Design review of the part built by this model. Coordinates are the model's own, in mm. A direction names the side the tool comes from. Coordinates: 2 decimals unless noted, no trailing zeros. Write each loop counter-clockwise with the first axis right and the second up, starting at its lowest first coordinate (ties: lowest second). Pieces come first, ordered by that corner, then holes. Notation, with made-up numbers: (44.25, 19.25) - (66.25, 19.25) arc R16 ccw to (66.25, 41.25) - close; hole circle Ø6 at (52, -20). An arc over 180 degrees is marked (long way). One line per item, written item: value.
Autodesk Inventor part; units mm, degrees
ref_plane "Arbeitsebene1" through (53.5, 2, 88) normal (1, 0, 0) x (0, 0, -1)
ref_plane "Arbeitsebene7" through (18, 0, -130) normal (0, 0, -1) x (-1, 0, 0)
ref_plane "YZ Plane" through (0, 0, 0) normal (1, 0, 0) x (0, 1, 0)
sketch "Skizze1" plane through (0, 0, 0) normal (0, 1, 0) x (-1, 0, 0)
  line L0 (53, 90) -> (53, 20)
  line L1 (53, 20) -> (18, 0)
  line L2 (18, 0) -> (-18, 0)
  line L3 (-18, 0) -> (-53, 20)
  line L4 (-53, 20) -> (-53, 90)
  line L5 (-53, 90) -> (-39.5, 90)
  line L6 (-39.5, 90) -> (-39.5, 30)
  line L7 (-39.5, 30) -> (-15, 15)
  line L8 (-15, 15) -> (15, 15)
  line L9 (15, 15) -> (39.5, 30)
  line L10 (39.5, 30) -> (39.5, 90)
  line L11 (39.5, 90) -> (53, 90)
  line L12 (0, -234) -> (0, 144) construction
  point P0 (0, 0)
  dimension "d0" = 79
  dimension "d1" = 13.5
  dimension "d2" = 13.5
  dimension "d3" = 90
  dimension "d5" = 60
  dimension "d6" = 15
  dimension "d7" = 60
  dimension "d8" = 70
  dimension "d9" = 70
  dimension "d12" = 15
  dimension "d13" = 15
  dimension "d14" = 18
  dimension "d15" = 18
extrude "Extrusion1" add sketch "Skizze1" along normal blind 20
sketch "Skizze2" plane through (18, 0, 0) normal (0, 0, -1) x (-1, 0, 0)
  line L0 (57.5, 20) -> (33, 20) construction
  line L1 (8.5, 0) -> (27.5, 0)
  line L2 (27.5, 0) -> (27.5, 20)
  line L3 (27.5, 20) -> (8.5, 20)
  line L4 (8.5, 20) -> (8.5, 0)
  line L5 (18, -4) -> (18, 24) construction
  line L6 (0, 0) -> (36, 0) construction
  point P0 (18, 0)
  point P1 (18, 0)
  point P2 (18, 20)
  dimension "d75" = 19
extrude "Extrusion2" add sketch "Skizze2" along normal blind 180
ref_plane "Arbeitsebene1" through (53.5, 2, 88) normal (1, 0, 0) x (0, 0, -1)
sketch "Skizze3" plane through (53, 0, 90) normal (1, 0, 0) x (0, 0, -1)
  line L0 (0, 10) -> (14, 10) construction
  line L1 (0, 0) -> (0, 20) construction
  circle A0 centre (14, 10) radius 6
  dimension "d44" = 14
  dimension "d87" = 12
extrude "Extrusion3" cut sketch "Skizze3" against normal through all
ref_plane "Arbeitsebene5" through (18, 0, -160) normal (0, 0, -1) x (-1, 0, 0)
ref_plane "Arbeitsebene6" through (18, 0, -100) normal (0, 0, -1) x (-1, 0, 0)
ref_plane "Arbeitsebene7" through (18, 0, -130) normal (0, 0, -1) x (-1, 0, 0)
sketch "Skizze13" plane through (9.5, 0, 0) normal (1, 0, 0) x (0, 0, -1)
  line L0 (160, 24) -> (160, -4) construction
  line L1 (100, 24) -> (100, -4) construction
  line L2 (180, 0) -> (180, 20) construction
  line L3 (180, 10) -> (100, 10) construction
  point P0 (0, 0)
  point P1 (160, 10)
hole "Bohrung2" at (9.5, 10, -100) at (9.5, 10, -160) direction (-1, 0, 0) diameter 8.376 end through all
sketch "Skizze11" plane through (0, 20, 0) normal (0, 1, 0) x (1, 0, 0)
  line L0 (9.5, 0) -> (18, 0)
  line L1 (18, 0) -> (18, 61.5)
  line L2 (9.5, 70) -> (9.5, 0)
  line L3 (-9.5, 0) -> (-9.5, 180)
  line L4 (-9.5, 0) -> (-18, 0)
  line L5 (-18, 0) -> (-18, 61.5)
  line L6 (-9.5, 70) -> (-9.5, 0)
  arc A0 (9.5, 70) -> (18, 61.5) centre (18, 70) ccw
  arc A1 (-18, 61.5) -> (-9.5, 70) centre (-18, 70) ccw
  point P0 (0, 0)
  point P1 (-9.5, 70)
  dimension "d80" = 70
  dimension "d81" = 70
extrude "Extrusion7" add sketch "Skizze11" against normal up to surface (20 mm away)
sketch "Skizze12" plane through (18, 0, -180) normal (0, 0, -1) x (-1, 0, 0)
  line L0 (27.5, 20) -> (8.5, 20) construction
  point P0 (18, 0)
  dimension "Gabel_FixierungPart_Width" = 19
chamfer "Fase1" distance 1.25 angle 45 4 edges at (9.5, 10, -155.812) (9.5, 10, -95.812) (-9.5, 10, -155.812) (-9.5, 10, -95.812)
chamfer "Fase2" distance 0.5 angle 45 4 edges at (53, 10, 82) (39.5, 10, 82) (-53, 10, 82) (-39.5, 10, 82)
equation "\"d1\" = d2"
equation "\"d75\" = ParallelMecha_Contact_Dist - 2 * Gabel_FixationShaft_Contact_Thickness"
equation "\"d81\" = d80"
equation "\"Fixation_dist2\" = -Total_Bearing_Hole_Dist"
properties part number "Adaptationhorizontalachse" material "Aluminum 6061-AHC"
1. Wall thickness on line 1 along Y through (x, z) = (-49, 76); line 2 along Y through (x, z) = (-4, -160); line 3 along X through (y, z) = (3, -82): over which ranges is each line inside the solid? List them lowest first.
Answer block:
line 1: y = 0 to 4, 16 to 20
line 2: y = 0 to 5.81, 14.19 to 20
line 3: x = -9.5 to 9.5
2. Consider section D-D, the plane z = -73. Write out the cut boundary in (x, y).
Answer block:
outline: (-9.5, 0) - (9.5, 0) - (9.5, 20) - (-9.5, 20) - close
3. Consider section B-B, the plane z = 76. Write out the cut boundary in (x, y).
Answer block:
outline: (-53, 0) - (-39.5, 0) - (-39.5, 3.5) - (-40, 4) - (-52.5, 4) - (-53, 3.5) - close; (-53, 16.5) - (-52.5, 16) - (-40, 16) - (-39.5, 16.5) - (-39.5, 20) - (-53, 20) - close; (39.5, 0) - (53, 0) - (53, 3.5) - (52.5, 4) - (40, 4) - (39.5, 3.5) - close; (39.5, 16.5) - (40, 16) - (52.5, 16) - (53, 16.5) - (53, 20) - (39.5, 20) - close
4. Mouldability with a two-part tool opening along X and no side actions: class faces 4 (the face through (-39.5, 10, 60)), 5 (the face through (-18, 10, -30)), 6 (the face through (-27.078, 9.86, 22.395)), 7 (the face through (46, 10, 82)) as released by +X, released by -X, zero draft, split by the parting line, or undercut.
Answer block:
face 4: undercut
face 5: released by -X
face 6: undercut
face 7: zero draft
5. For faces 1 (the face through (9.5, 10, -124)), 2 (the face through (39.5, 10, 60)), 3 (the face through (4, 0, -24)), list the 3-axis set-ups (+Z, -Z, +X, -X, +Y, -Y) from which the entire face can be reached by the end or side of a thin tool; tool diameter is ignored.
Answer block:
face 1: -Z, +X, +Y, -Y
face 2: +Z, +Y, -Y
face 3: +Z, -Z, +X, -X, -Y
6. Consider section C-C, the plane x = -45.5. Write out the cut boundary in (y, z), then the cut area to 3 significant figures.
Answer block:
outline: (0, 15.71) - (20, 15.71) - (20, 90) - (0, 90) - close; hole circle Ø12 at (10, 76)
area: 1,370 mm^2
7. Insertion check: pin 1 Ø11 at (y, z) = (10, 76) entering from -X; pin 2 Ø10 at (y, z) = (14, -28.5) entering from +X; pin 3 Ø10 at (x, y) = (-19.5, 5) entering from +Z; pin 4 Ø1 at (x, y) = (-37.5, 17) entering from +Z. Each pin has a flat end and moves straight along its axis. Give the tip position at first contact, or say it passes through.
Answer block:
pin 1: passes through
pin 2: stops at x = 18
pin 3: stops at z = 20.82
pin 4: stops at z = 29.08
8. Consider section A-A, the plane z = -160. Write out the cut boundary in (x, y).
Answer block:
outline: (-9.5, 0) - (9.5, 0) - (9.5, 4.56) - (8.25, 5.81) - (-8.25, 5.81) - (-9.5, 4.56) - close; (-9.5, 15.44) - (-8.25, 14.19) - (8.25, 14.19) - (9.5, 15.44) - (9.5, 20) - (-9.5, 20) - close
